Model file for the job. Use its own axes, mm. Face numbers are marked on the shaded views. A direction names the side the tool comes from. Give positions to 0.01 mm unless a question says otherwise; leave off trailing zeros. Write each loop counter-clockwise with the first axis right and the second up, starting at its lowest first coordinate (ties: lowest second). Pieces come first, ordered by that corner, then holes. Notation, with made-up numbers: M 57,49.25 L 65,49.25 A20 ccw 65,83.25 Z; hole C 26.5,58.5 d6. An arc over 180 degrees is marked long. Answer as a JSON object with one key per item and string values. Group by question number.
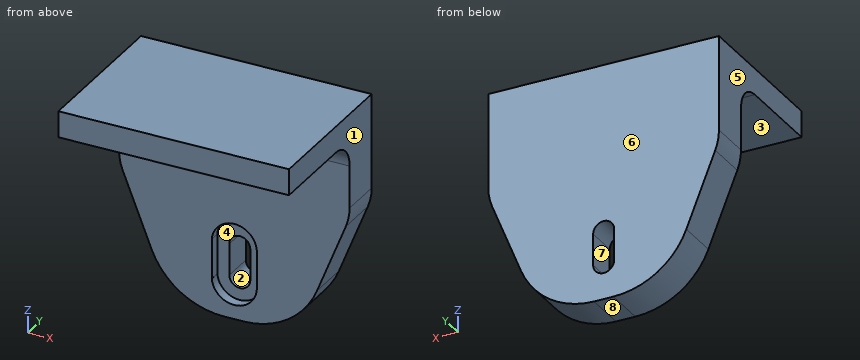
```python
from build123d import *

# Parameters (mm, degrees)
BOX009_W                  = 8.6
BOX009_H                  = 14
BOX009_DEPTH              = 7.6
CYLINDER017_R             = 4.3
CYLINDER017_DEPTH         = 10
CYLINDER016_R             = 4.3
CYLINDER016_DEPTH         = 10
CYLINDER018_R             = 2
CYLINDER018_DEPTH         = 10
CYLINDER019_R             = 4.25
CYLINDER019_DEPTH         = 10
CYLINDER015_R             = 2
CYLINDER015_DEPTH         = 10
BOX008_W                  = 4
BOX008_H                  = 16
BOX008_DEPTH              = 6
BOX010_W                  = 15
BOX010_H                  = 8
BOX010_DEPTH              = 10
CYLINDER013_R             = 2
CYLINDER013_DEPTH         = 10
CYLINDER014_R             = 4.25
CYLINDER014_DEPTH         = 10
FUSION013_PLACEMENT_ANGLE = 180
CYLINDER010_R             = 4.25
CYLINDER010_DEPTH         = 10
CYLINDER011_R             = 2
CYLINDER011_DEPTH         = 10
CYLINDER012_R             = 4.25
CYLINDER012_DEPTH         = 10
EXTRUDE001_DEPTH          = 8
BOX007_W                  = 24
BOX007_H                  = 8
BOX007_DEPTH              = 45
BOX006_W                  = 44
BOX006_H                  = 8
BOX006_DEPTH              = 15
BOX005_W                  = 44
BOX005_H                  = 30
BOX005_DEPTH              = 5
FILLET003_R               = 5
FILLET005_R               = 15
FILLET004_R               = 10
CHAMFER004_SIZE           = 2.2
CHAMFER005_SIZE           = 2.2


with BuildPart() as cube009:
    # Box009 → Box009 (new body)
    with BuildSketch(Plane(origin=(17.7, 59, -33.3), x_dir=(1, 0, 0), z_dir=(0, 0, 1))):
        with Locations((4.3, 7)):
            Rectangle(BOX009_W, BOX009_H)
    extrude(amount=BOX009_DEPTH)


with BuildPart() as cylinder017:
    # Cylinder017 → Cylinder017 (new body)
    with BuildSketch(Plane(origin=(22, 73, -26), x_dir=(1, 0, 0), z_dir=(0, -1, 0))):
        Circle(CYLINDER017_R)
    extrude(amount=CYLINDER017_DEPTH)


with BuildPart() as obj1:
    # Cylinder016 → Cylinder016 (new body)
    with BuildSketch(Plane(origin=(22, 73, -33), x_dir=(1, 0, 0), z_dir=(0, -1, 0))):
        Circle(CYLINDER016_R)
    extrude(amount=CYLINDER016_DEPTH)

    # Fusion017: union Cube009, Cylinder017
    add(cube009.part)
    add(cylinder017.part)


with BuildPart() as obj1_1:
    # Fusion017 placement: moved
    add(obj1.part.moved(Location((0, 1, 0))))


with BuildPart() as cylinder018:
    # Cylinder018 → Cylinder018 (new body)
    with BuildSketch(Plane(origin=(22, 80, -33), x_dir=(1, 0, 0), z_dir=(0, -1, 0))):
        Circle(CYLINDER018_R)
    extrude(amount=CYLINDER018_DEPTH)


with BuildPart() as fusion018:
    # Cylinder019 → Cylinder019 (new body)
    with BuildSketch(Plane(origin=(22, 89, -33), x_dir=(1, 0, 0), z_dir=(0, -1, 0))):
        Circle(CYLINDER019_R)
    extrude(amount=CYLINDER019_DEPTH)

    # Fusion018: union Cylinder018
    add(cylinder018.part)


with BuildPart() as cylinder015:
    # Cylinder015 → Cylinder015 (new body)
    with BuildSketch(Plane(origin=(22, 80, -27), x_dir=(1, 0, 0), z_dir=(0, -1, 0))):
        Circle(CYLINDER015_R)
    extrude(amount=CYLINDER015_DEPTH)


with BuildPart() as obj2:
    # Box008 → Box008 (new body)
    with BuildSketch(Plane(origin=(20, 69, -33), x_dir=(1, 0, 0), z_dir=(0, 0, 1))):
        with Locations((2, 8)):
            Rectangle(BOX008_W, BOX008_H)
    extrude(amount=BOX008_DEPTH)

    # Fusion016: union Cylinder015
    add(cylinder015.part)

    # Fusion019: union Fusion018
    add(fusion018.part)


with BuildPart() as obj2_1:
    # Fusion019 placement: moved
    add(obj2.part.moved(Location((0, 2, 0))))


with BuildPart() as cube010:
    # Box010 → Box010 (new body)
    with BuildSketch(Plane(origin=(14, 72, -38), x_dir=(1, 0, 0), z_dir=(0, 0, 1))):
        with Locations((7.5, 4)):
            Rectangle(BOX010_W, BOX010_H)
    extrude(amount=BOX010_DEPTH)


with BuildPart() as cylinder013:
    # Cylinder013 → Cylinder013 (new body)
    with BuildSketch(Plane(origin=(22, 80, -33), x_dir=(1, 0, 0), z_dir=(0, -1, 0))):
        Circle(CYLINDER013_R)
    extrude(amount=CYLINDER013_DEPTH)


with BuildPart() as fusion013:
    # Cylinder014 → Cylinder014 (new body)
    with BuildSketch(Plane(origin=(22, 89, -33), x_dir=(1, 0, 0), z_dir=(0, -1, 0))):
        Circle(CYLINDER014_R)
    extrude(amount=CYLINDER014_DEPTH)

    # Fusion013: union Cylinder013
    add(cylinder013.part)


with BuildPart() as fusion013_1:
    # Fusion013 placement: moved
    add(fusion013.part.moved(Location((0, 152, -66))).rotate(Axis((0, 152, -66), (1, 0, 0)), FUSION013_PLACEMENT_ANGLE))


with BuildPart() as cylinder010:
    # Cylinder010 → Cylinder010 (new body)
    with BuildSketch(Plane(origin=(22, 80, -33), x_dir=(1, 0, 0), z_dir=(0, -1, 0))):
        Circle(CYLINDER010_R)
    extrude(amount=CYLINDER010_DEPTH)


with BuildPart() as cylinder011:
    # Cylinder011 → Cylinder011 (new body)
    with BuildSketch(Plane(origin=(22, 80, -33), x_dir=(1, 0, 0), z_dir=(0, -1, 0))):
        Circle(CYLINDER011_R)
    extrude(amount=CYLINDER011_DEPTH)


with BuildPart() as fusion010:
    # Cylinder012 → Cylinder012 (new body)
    with BuildSketch(Plane(origin=(22, 89, -33), x_dir=(1, 0, 0), z_dir=(0, -1, 0))):
        Circle(CYLINDER012_R)
    extrude(amount=CYLINDER012_DEPTH)

    # Fusion010: union Cylinder011
    add(cylinder011.part)


with BuildPart() as extrude001:
    # Sketch001 (on Face11 of Fusion012) → Extrude001 (new body)
    with BuildSketch(Plane(origin=(0, 80, 0), x_dir=(-1, 0, 0), z_dir=(0, 1, 0))):
        Polygon((-44, -15), (-34, -40), (-34, -15), align=None)
        Polygon((-10, -15), (0, -15), (-10, -40), align=None)
    extrude(amount=-EXTRUDE001_DEPTH)


with BuildPart() as cube007:
    # Box007 → Box007 (new body)
    with BuildSketch(Plane(origin=(10, 72, -40), x_dir=(1, 0, 0), z_dir=(0, 0, 1))):
        with Locations((12, 4)):
            Rectangle(BOX007_W, BOX007_H)
    extrude(amount=BOX007_DEPTH)


with BuildPart() as cube006:
    # Box006 → Box006 (new body)
    with BuildSketch(Plane(origin=(0, 72, -15), x_dir=(1, 0, 0), z_dir=(0, 0, 1))):
        with Locations((22, 4)):
            Rectangle(BOX006_W, BOX006_H)
    extrude(amount=BOX006_DEPTH)


with BuildPart() as cut007:
    # Box005 → Box005 (new body)
    with BuildSketch(Plane(origin=(0, 50, 0), x_dir=(1, 0, 0), z_dir=(0, 0, 1))):
        with Locations((22, 15)):
            Rectangle(BOX005_W, BOX005_H)
    extrude(amount=BOX005_DEPTH)

    # Fusion014: union Cube006
    add(cube006.part)

    # Fillet003
    fillet003_edges = [cut007.edges().sort_by_distance(p)[0] for p in [
        (22, 72, 0),
    ]]
    fillet(fillet003_edges, radius=FILLET003_R)

    # Fusion012: union Cube007
    add(cube007.part)

    # Fusion015: union Extrude001
    add(extrude001.part)

    # Fillet005
    fillet005_edges = [cut007.edges().sort_by_distance(p)[0] for p in [
        (10, 76, -40),
        (34, 76, -40),
    ]]
    fillet(fillet005_edges, radius=FILLET005_R)

    # Fillet004
    fillet004_edges = [cut007.edges().sort_by_distance(p)[0] for p in [
        (44, 76, -15),
        (0, 76, -15),
    ]]
    fillet(fillet004_edges, radius=FILLET004_R)

    # Cut004: cut Fusion010
    add(fusion010.part, mode=Mode.SUBTRACT)

    # Chamfer004
    chamfer004_edges = [cut007.edges().sort_by_distance(p)[0] for p in [
        (20, 79, -33),
    ]]
    chamfer(chamfer004_edges, length=CHAMFER004_SIZE)

    # Fusion011: union Cylinder010
    add(cylinder010.part)

    # Cut005: cut Fusion013
    add(fusion013_1.part, mode=Mode.SUBTRACT)

    # Chamfer005
    chamfer005_edges = [cut007.edges().sort_by_distance(p)[0] for p in [
        (20, 73, -33),
    ]]
    chamfer(chamfer005_edges, length=CHAMFER005_SIZE)

    # Fusion020: union Cube010
    add(cube010.part)

    # Cut006: cut obj2
    add(obj2_1.part, mode=Mode.SUBTRACT)

    # Cut007: cut obj1
    add(obj1_1.part, mode=Mode.SUBTRACT)


solid = cut007.part
```
Q1. Slice it at C-C, the plane x = 13.5. Write the cut outline in (y, z), then the cut area to 3 significant figures.
Q2. Slice it at B-B, the plane z = -32. Write the cut outline in (x, y).
Q3. Wall check: L1, parallel to Y at x = 28, z = -37.5; L2, parallel to Z at x = 19, y = 54; L3, parallel to Y at x = 20.5, z = -25. Give the ranges that are in metal, low to high.
Q4. Slice it at D-D, the plane z = -9. Write the cut outline in (x, y).
Q5. Drop flat-ended pins along their axis: P1, Ø10, axis at x = 10.5, y = 57.5, coming from the -Z side; P2, Ø3, axis at y = 77.5, z = -29.5, coming from the -X side; P3, Ø4, axis at y = 70.5, z = -29.5, coming from the -X side; P4, Ø2.5, axis at x = 22.5, z = -33, coming from the -Y side. Give the stop position or say it passes through.
Q6. Two-plate mould, pull along Z, no slides. Class the marked faces 6, 7 and 8: +Z half, -Z half, draft (parallel to the pull), parting line (faces both ways), or undercut.
Q7. Slice it at A-A, the plane x = 22. Write the cut outline in (y, z).
Q8. 3-axis set-ups, long thin cutter, end or side, ignore diameter. For the marked faces 1, 2, 3, 4 and 5: which of +Z, -Z, +X, -X, +Y, -Y reach the whole face in a straight line?
Solved:
{
 "1": {"outline": "M 50,0 L 67,0 A5 cw 72,-5 L 72,-38.44 L 80,-38.44 L 80,5 L 50,5 Z", "area": "463 mm²"},
 "2": {"outline": "M 6.89,72 L 17.7,72 L 17.7,74 L 20,74 L 20,80 L 6.89,80 Z; M 24,74 L 26.3,74 L 26.3,72 L 37.11,72 L 37.11,80 L 24,80 Z"},
 "3": {"L1": "y = 72 to 80", "L2": "z = 0 to 5", "L3": "y = 74 to 80"},
 "4": {"outline": "M 0,72 L 44,72 L 44,80 L 0,80 Z"},
 "5": {"P1": "stops at z = 0", "P2": "stops at x = 5.2", "P3": "stops at x = 5.27", "P4": "passes through"},
 "6": {"face 6": "draft", "face 7": "undercut", "face 8": "-Z half"},
 "7": {"outline": "M 50,0 L 67,0 A5 cw 72,-5 L 72,-21.7 L 74,-21.7 L 74,-25 L 80,-25 L 80,5 L 50,5 Z; M 72,-40 L 80,-40 L 80,-35 L 74,-35 L 74,-37.3 L 72,-37.3 Z"},
 "8": {"face 1": "+Z, -Z, +X, +Y, -Y", "face 2": "+Y, -Y", "face 3": "-Z, +X, -X, -Y", "face 4": "-Y", "face 5": "+Z, -Z, -X, +Y, -Y"}
}
